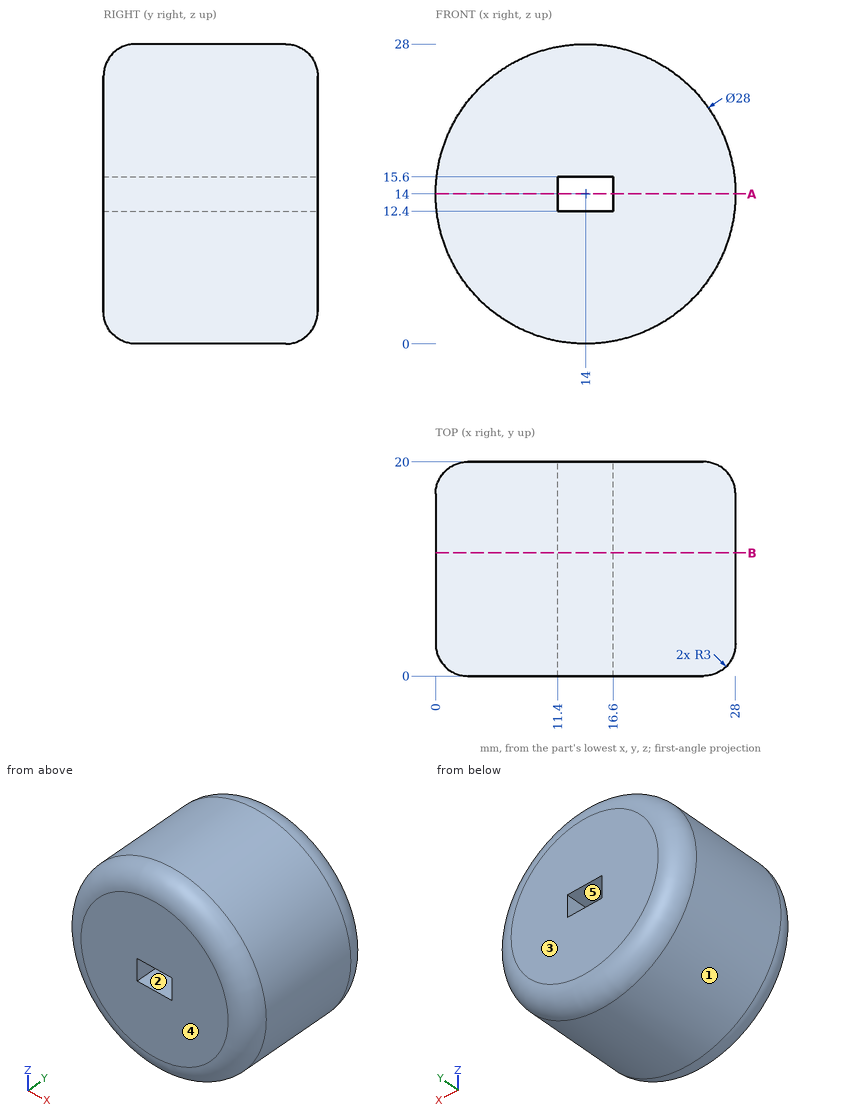
Drawing for the job (mm, zero at the part's lowest x, y, z). A direction names the side the tool comes from. Round coordinates to 2 decimals unless told otherwise and drop trailing zeros. Loops run counter-clockwise (first coordinate to the right, second up) from the corner with the lowest first, then second, coordinate; pieces in that order, holes last.
1. Mould opens along Z. For the marked faces 1, 2 and 3 say: +Z half, -Z half, draft (parallel to the pull), parting line (faces both ways), or undercut.
Check values:
face 1: parting line
face 2: undercut
face 3: draft
2. Wall check: probe 1 along Z at (x, y) = (20, 15.5); probe 2 along Z at (x, y) = (14.5, 12.25); probe 3 along X at (y, z) = (7.25, 5). Give the ranges that are in metal, low to high.
Check values:
probe 1: z = 1.35 to 26.65
probe 2: z = 0.01 to 12.4, 15.6 to 27.99
probe 3: x = 3.28 to 24.72
3. Band-saw the part on B-B, the plane y = 11.5. List the corners of the cut face in (x, z), and give its area (3 significant figures).
Check values:
outline: circle Ø28 at (14, 14); hole (11.4, 12.4) - (16.6, 12.4) - (16.6, 15.6) - (11.4, 15.6) - close
area: 599 mm2
4. Tool access for the marked faces 4 and 5: list every direction of +Z, -Z, +X, -X, +Y, -Y with a clear straight run to the whole face (end or side of a thin tool).
Check values:
face 4: +Z, -Z, +X, -X, -Y
face 5: +Y, -Y
5. Drop flat-ended pins along their axis: P1, Ø5, axis at x = 9.5, y = 9.5, coming from the -Z side; P2, Ø8, axis at y = 10.5, z = 5.5, coming from the +X side; P3, Ø5, axis at y = 13, z = 6.5, coming from the +X side. Give the stop position or say it passes through.
Check values:
P1: stops at z = 0.14
P2: stops at x = 27.26
P3: stops at x = 27.08
6. Band-saw the part on A-A, the plane z = 14. List the corners of the cut face in (x, y), and give its area (3 significant figures).
Check values:
outline: (0, 3) arc R3 ccw to (3, 0) - (11.4, 0) - (11.4, 20) - (3, 20) arc R3 ccw to (0, 17) - close; (16.6, 0) - (25, 0) arc R3 ccw to (28, 3) - (28, 17) arc R3 ccw to (25, 20) - (16.6, 20) - close
area: 448 mm2
